Input: part model. Units: mm. Frame: model coordinates. Give positions to 0.01 mm unless a question says otherwise; leave off trailing zeros. Loops run counter-clockwise (first coordinate to the right, second up) from the corner with the lowest first, then second, coordinate; pieces in that order, holes last. Notation, with made-up numbers: M 22,34 L 35,34 A25 cw 35,56 Z; hole C 12,52.5 d9. An arc over 180 degrees is marked long. Use a Markdown table: item, result. Add a question column.
from build123d import *

# Parameters (mm, degrees)
SKETCH1_W           = 299.398126018
SKETCH1_H           = 56.59882
SKETCH1_R           = 2.625
BOSS_EXTRUDE1_DEPTH = 3.175
SKETCH2_R           = 1
CUT_EXTRUDE1_DEPTH  = 4.175
SKETCH3_R           = 1.778
CUT_EXTRUDE2_DEPTH  = 4.175
CUT_EXTRUDE3_DEPTH  = 4.175


with BuildPart() as part:
    # Sketch1 → Boss-Extrude1 (new body)
    with BuildSketch(Plane.XY):
        with Locations((162.727004442, 111.211757818)):
            Rectangle(SKETCH1_W, SKETCH1_H)
        with Locations((286.266607451, 133.161167818)):
            Circle(SKETCH1_R, mode=Mode.SUBTRACT)
        with Locations((286.266607451, 89.262347818)):
            Circle(SKETCH1_R, mode=Mode.SUBTRACT)
        with Locations((39.187401433, 133.161167818)):
            Circle(SKETCH1_R, mode=Mode.SUBTRACT)
        with Locations((39.187401433, 89.262347818)):
            Circle(SKETCH1_R, mode=Mode.SUBTRACT)
    extrude(amount=BOSS_EXTRUDE1_DEPTH)

    # Sketch2 → Cut-Extrude1 (cut, through all)
    with BuildSketch(Plane.XY.offset(3.175)):
        with Locations((280.504156768, 117.824340674)):
            Circle(SKETCH2_R)
        with Locations((280.335334394, 99.825132385)):
            Circle(SKETCH2_R)
        with Locations((262.504948479, 117.993163047)):
            Circle(SKETCH2_R)
        with Locations((262.336126106, 99.993954759)):
            Circle(SKETCH2_R)
        with Locations((62.845741433, 117.909047818)):
            Circle(SKETCH2_R)
        with Locations((62.845741433, 99.909047818)):
            Circle(SKETCH2_R)
        with Locations((44.845741433, 117.909047818)):
            Circle(SKETCH2_R)
        with Locations((44.845741433, 99.909047818)):
            Circle(SKETCH2_R)
    extrude(amount=-CUT_EXTRUDE1_DEPTH, mode=Mode.SUBTRACT)

    # Sketch3 → Cut-Extrude2 (cut, through all)
    with BuildSketch(Plane.XY.offset(3.175)):
        with Locations((76.695557497, 117.909047818)):
            Circle(SKETCH3_R)
        with Locations((76.695557497, 99.909047818)):
            Circle(SKETCH3_R)
        with Locations((102.895189625, 117.909047818)):
            Circle(SKETCH3_R)
        with Locations((102.895189625, 99.909047818)):
            Circle(SKETCH3_R)
        with Locations((248.758451386, 99.909047818)):
            Circle(SKETCH3_R)
        with Locations((222.558819258, 99.909047818)):
            Circle(SKETCH3_R)
        with Locations((222.558819258, 117.909047818)):
            Circle(SKETCH3_R)
        with Locations((248.758451386, 117.909047818)):
            Circle(SKETCH3_R)
        with Locations((162.727004442, 91.563754554)):
            Circle(SKETCH3_R)
    extrude(amount=-CUT_EXTRUDE2_DEPTH, mode=Mode.SUBTRACT)

    # Sketch5 → Cut-Extrude3 (cut, through all)
    with BuildSketch(Plane.XY.offset(3.175)):
        with BuildLine():
            Line((53.845741433, 116.163287818), (13.027941433, 116.163287818))
            Line((13.027941433, 116.163287818), (13.027941433, 101.654807818))
            Line((13.027941433, 101.654807818), (53.845741433, 101.654807818))
            ThreePointArc((53.845741433, 101.654807818), (61.099981433, 108.909047818), (53.845741433, 116.163287818))
        make_face()
        with BuildLine():
            Line((271.608267451, 101.654807818), (312.426067451, 101.654807818))
            Line((312.426067451, 101.654807818), (312.426067451, 116.163287818))
            Line((312.426067451, 116.163287818), (271.608267451, 116.163287818))
            ThreePointArc((271.608267451, 116.163287818), (264.354027451, 108.909047818), (271.608267451, 101.654807818))
        make_face()
    extrude(amount=-CUT_EXTRUDE3_DEPTH, mode=Mode.SUBTRACT)


solid = part.part
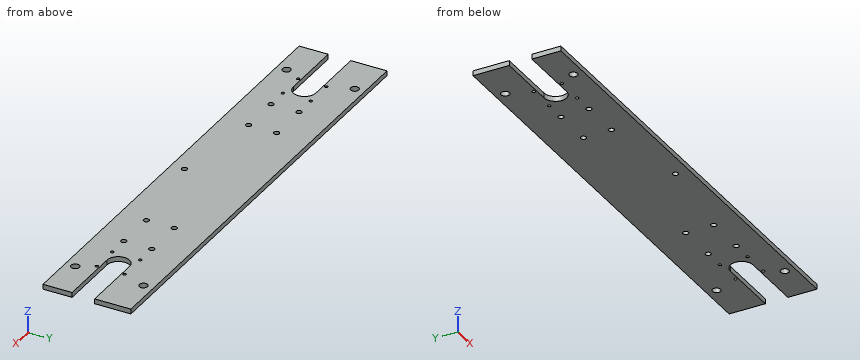
1) Section query A-A, the plane z = 0.5. State how many separate pieces and enclosed holes the cut face has, and give its area (3 significant figures).
2) Section query B-B, the plane y = 104.5. Return the cut outline in (x, z) (3 decimals), and give its area (3 significant figures).
3) Ray query, line 1 (Y direction, x = 37.5, z = 1.2); line 2 (Y direction, x = 299, z = 1.4); line 3 (X direction, y = 110, z = 1). Return the intervals inside material, ascending. Write a range as [from, to].
Entries:
| question | item | result |
|---|---|---|
| 1 | separate pieces | 1 |
| 1 | enclosed holes | 21 |
| 1 | area | 15,400 mm² |
| 2 | outline | M 59.606,0 L 265.848,0 L 265.848,3.175 L 59.606,3.175 Z |
| 2 | area | 655 mm² |
| 3 | line 1 | y = [82.91, 87.25], [91.27, 101.65], [116.16, 131.15], [135.17, 139.51] |
| 3 | line 2 | y = [82.91, 101.65], [116.16, 139.51] |
| 3 | line 3 | x = [61.02, 264.44] |
